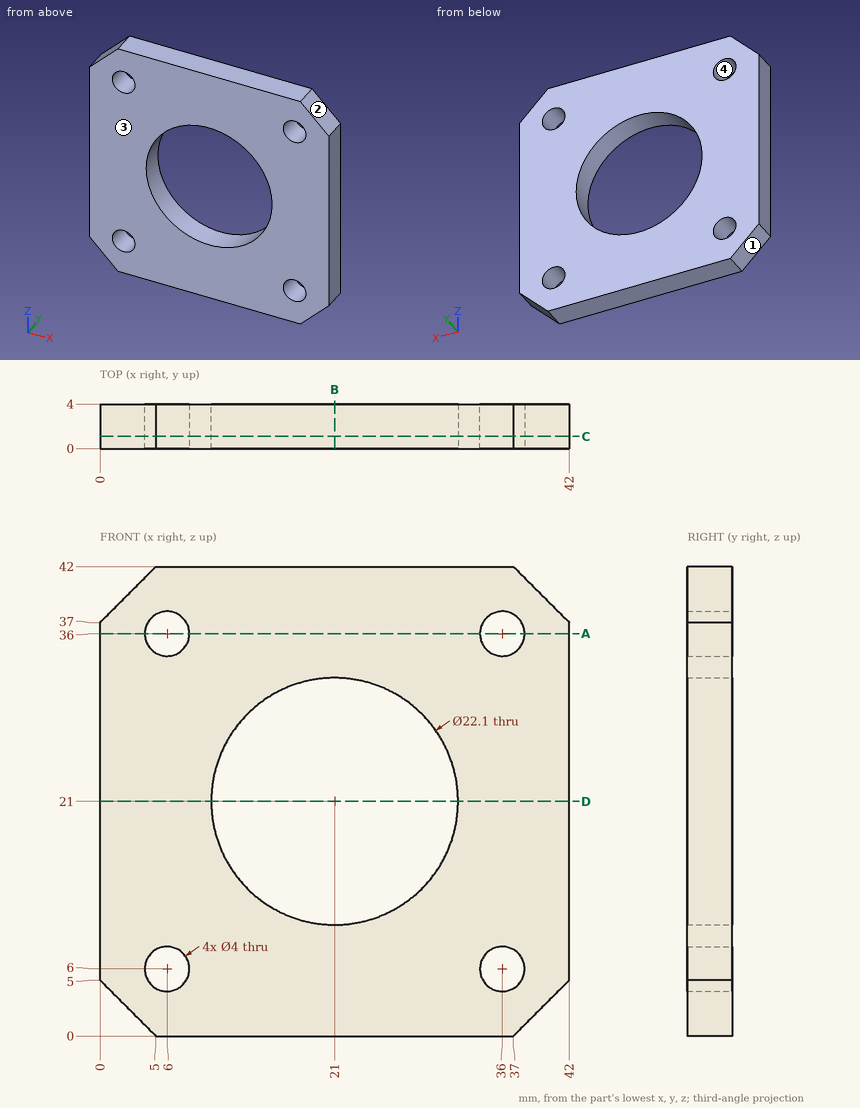
Can you work these out from the drawing? Everything is in mm from the part's minimum corner. Round coordinates to 2 decimals unless told otherwise and drop trailing zeros. Write each loop counter-clockwise with the first axis right and the second up, starting at its lowest first coordinate (ties: lowest second). Pieces come first, ordered by that corner, then holes. Notation, with made-up numbers: (-35, 8) - (-6, 8) arc R17 ccw to (-6, 17) - close; hole circle Ø6 at (44, 37). An arc over 180 degrees is marked (long way). Put each result on its own line as item: value. Start each with the question number.
(1) Thinking about a two-plate mould opening in X: for the marked faces 1, 2, 3 and 4, which applies, released by +X, released by -X, zero draft, split by the parting line, or undercut?
(2) I want a section at D-D, the plane z = 21. Please give me the cut outline in (x, y), plus the area to 3 significant figures.
(3) I want a section at B-B, the plane x = 21. Please give me the cut outline in (y, z), plus the area to 3 significant figures.
(4) I want a section at C-C, the plane y = 1.1. Please give me the cut outline in (x, z).
(5) I want a section at A-A, the plane z = 36. Please give me the cut outline in (x, y), plus the area to 3 significant figures.
(6) I need wall thicknesses on probe 1 along Z at (x, y) = (36, 1.3); probe 2 along Z at (x, y) = (30, 3.45); probe 3 along X at (y, z) = (0.65, 5.5). Which ranges of each line are inside material? Lowest first, please.
(7) Will this pin go through, and if not, where does the flat tip stop? pin 1 (2.5 mm diameter, centred on x = 6, z = 6, fed in from +Y).
Here are the results:
1. face 1: released by -X
1. face 2: released by +X
1. face 3: zero draft
1. face 4: undercut
2. outline: (0, 0) - (9.95, 0) - (9.95, 4) - (0, 4) - close; (32.05, 0) - (42, 0) - (42, 4) - (32.05, 4) - close
2. area: 79.6 mm^2
3. outline: (0, 0) - (4, 0) - (4, 9.95) - (0, 9.95) - close; (0, 32.05) - (4, 32.05) - (4, 42) - (0, 42) - close
3. area: 79.6 mm^2
4. outline: (0, 5) - (5, 0) - (37, 0) - (42, 5) - (42, 37) - (37, 42) - (5, 42) - (0, 37) - close; hole circle Ø4 at (6, 6); hole circle Ø4 at (6, 36); hole circle Ø22.1 at (21, 21); hole circle Ø4 at (36, 6); hole circle Ø4 at (36, 36)
5. outline: (0, 0) - (4, 0) - (4, 4) - (0, 4) - close; (8, 0) - (34, 0) - (34, 4) - (8, 4) - close; (38, 0) - (42, 0) - (42, 4) - (38, 4) - close
5. area: 136 mm^2
6. probe 1: z = 0 to 4, 8 to 34, 38 to 42
6. probe 2: z = 0 to 14.59, 27.41 to 42
6. probe 3: x = 0 to 4.06, 7.94 to 34.06, 37.94 to 42
7. pin 1: passes through
